Design review of the part shown in the three views and the two pictorial views. Dimensions are in mm from the part's minimum x, y and z. Round coordinates to 2 decimals unless told otherwise and drop trailing zeros. Loops run counter-clockwise (first coordinate to the right, second up) from the corner with the lowest first, then second, coordinate; pieces in that order, holes last. Notation, with made-up numbers: (0, -31.5) -> (44, -31.5) arc R31 cw to (44, 0.5) -> close; hole circle Ø4 at (49, 83). An arc over 180 degrees is marked (long way). Use a Markdown table: item, result. Add a question column.
1) Consider section C-C on x = 135.5. Give the boundary of the cut face in (y, z).
2) Mouldability with a two-part tool opening along Y and no side actions: class the marked faces 1 and 2 as released by +Y, released by -Y, zero draft, split by the parting line, or undercut.
3) Consider section A-A on z = 147. Give the boundary of the cut face in (x, y), plus the area to 3 significant figures.
4) Consider section D-D on z = 20. Give the boundary of the cut face in (x, y) (1 decimal), plus the area to 3 significant figures.
5) Insertion check: pin 1 (5 mm diameter, centred on x = 278.5, y = 3.5, fed in from +Z); pin 2 (2 mm diameter, centred on x = 271.5, z = 91.5, fed in from -Y); pin 3 (5 mm diameter, centred on x = 226.5, y = 8, fed in from +Z); pin 4 (5 mm diameter, centred on y = 3.5, z = 153, fed in from -X). Each pin has a flat end and moves straight along its axis. Give the tip position at first contact, or say it passes through.
6) Wall thickness on probe 1 along X at (y, z) = (1.25, 144); probe 2 along Z at (x, y) = (159, 6.5); probe 3 along X at (y, z) = (9.75, 32) (1 decimal): over which ranges is each line inside the solid? List them lowest first.
7) Consider section B-B on y = 3. Give the boundary of the cut face in (x, z) (1 decimal).
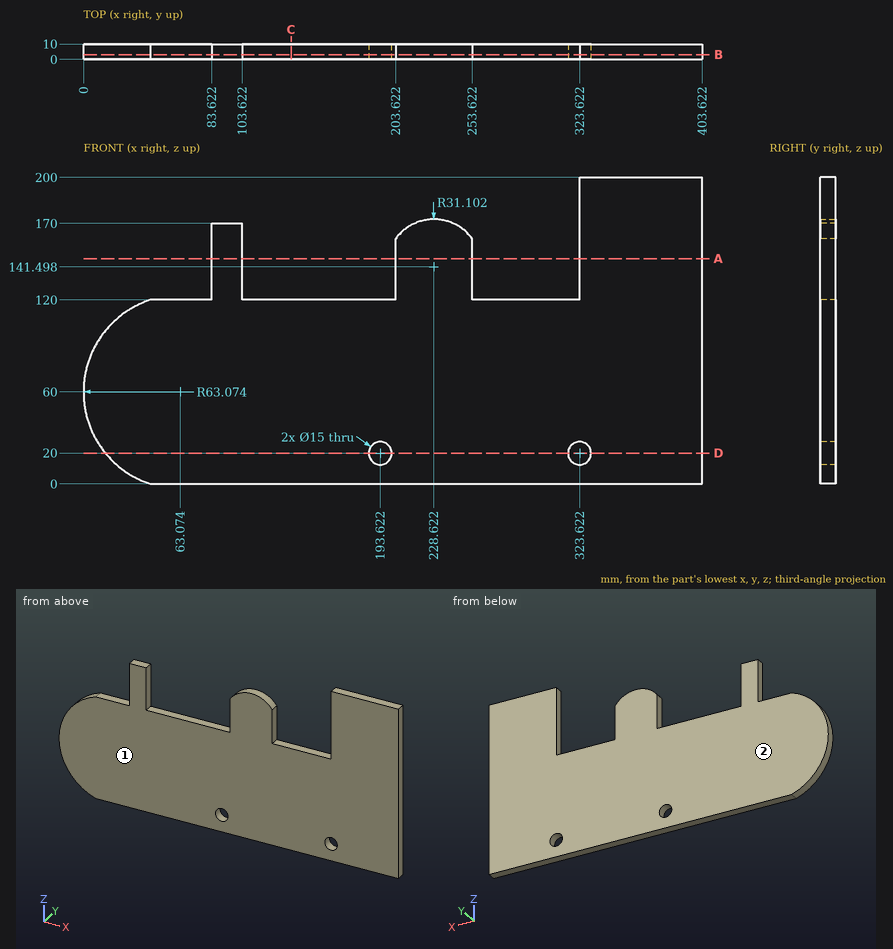
Result set:
| question | item | result |
|---|---|---|
| 1 | outline | (0, 0) -> (10, 0) -> (10, 120) -> (0, 120) -> close |
| 2 | face 1 | released by -Y |
| 2 | face 2 | released by +Y |
| 3 | outline | (83.62, 0) -> (103.62, 0) -> (103.62, 10) -> (83.62, 10) -> close; (203.62, 0) -> (253.62, 0) -> (253.62, 10) -> (203.62, 10) -> close; (323.62, 0) -> (403.62, 0) -> (403.62, 10) -> (323.62, 10) -> close |
| 3 | area | 1,500 mm2 |
| 4 | outline | (14.3, 0) -> (186.1, 0) -> (186.1, 10) -> (14.3, 10) -> close; (201.1, 0) -> (316.1, 0) -> (316.1, 10) -> (201.1, 10) -> close; (331.1, 0) -> (403.6, 0) -> (403.6, 10) -> (331.1, 10) -> close |
| 4 | area | 3,590 mm2 |
| 5 | pin 1 | z = 120 |
| 5 | pin 2 | y = 0 |
| 5 | pin 3 | z = 172.6 |
| 5 | pin 4 | x = 83.62 |
| 6 | probe 1 | 83.62 to 103.62, 203.62 to 253.62, 323.62 to 403.62 |
| 6 | probe 2 | 0 to 120 |
| 6 | probe 3 | 6.6 to 403.6 |
| 7 | outline | (43.6, 0) -> (403.6, 0) -> (403.6, 200) -> (323.6, 200) -> (323.6, 120) -> (253.6, 120) -> (253.6, 160) arc R31.1 ccw to (203.6, 160) -> (203.6, 120) -> (103.6, 120) -> (103.6, 170) -> (83.6, 170) -> (83.6, 120) -> (43.6, 120) arc R63.1 ccw to start; hole circle Ø15 at (193.6, 20); hole circle Ø15 at (323.6, 20) |
